Input: part model. Units: mm. Frame: model coordinates. A direction names the side the tool comes from. Give positions to 0.01 mm unless a question says otherwise; leave off trailing zeros. Write each loop counter-clockwise with the first axis right and the second up, starting at its lowest first coordinate (ties: lowest second). Pieces come first, ordered by that corner, then holes. Notation, with made-up numbers: (-30, -20) - (1, -20) arc R30 ccw to (1, 9) - close; hole circle Ø8 at (82, 38.5). An arc over 180 degrees is marked (long way). Answer as CSV lines item,"result". Start each with the question number.
from build123d import *

# Parameters (mm, degrees)
SKETCH056_R     = 1.05
PAD039_DEPTH    = 2
SKETCH057_W     = 10
SKETCH057_H     = 4
PAD040_DEPTH    = 10
SKETCH058_R     = 1.75
POCKET009_DEPTH = 4.001


with BuildPart() as part:
    # Sketch056 → Pad039 (new body)
    with BuildSketch(Plane.YZ):
        Polygon((-21.25, 67), (-16.25, 67), (-16.25, 39), (16.25, 39), (16.25, 67), (21.25, 67), (21.25, 34), (5, 34), (5, 4), (-5, 4), (-5, 34), (-21.25, 34), align=None)
        with Locations((-18.75, 60.75)):
            Circle(SKETCH056_R, mode=Mode.SUBTRACT)
        with Locations((-18.75, 45.25)):
            Circle(SKETCH056_R, mode=Mode.SUBTRACT)
        with Locations((18.75, 45.25)):
            Circle(SKETCH056_R, mode=Mode.SUBTRACT)
        with Locations((18.75, 60.75)):
            Circle(SKETCH056_R, mode=Mode.SUBTRACT)
    extrude(amount=PAD039_DEPTH)

    # Sketch057 (on Face18 of Pad039) → Pad040 (join)
    with BuildSketch(Plane.YZ.offset(2)):
        with Locations((0, 6)):
            Rectangle(SKETCH057_W, SKETCH057_H)
    extrude(amount=PAD040_DEPTH)

    # Sketch058 (on Face19 of Pad040) → Pocket009 (cut, through all)
    with BuildSketch(Plane(origin=(0, 0, 8), x_dir=(0, -1, 0), z_dir=(0, 0, 1))):
        with Locations((0, 7)):
            Circle(SKETCH058_R)
    extrude(amount=-POCKET009_DEPTH, mode=Mode.SUBTRACT)


with BuildPart() as part_1:
    # Body013 placement: moved
    add(part.part.moved(Location((41, 0, 0))))


solid = part_1.part
1) Contact query for flat-ended pins moving along their axis: P1, Ø1, axis at x = 42, y = -16.5, coming from the -Z side; P2, Ø5, axis at x = 44, z = 25.5, coming from the +Y side; P3, Ø1, axis at x = 42, y = -3, coming from the +Z side. Output: stop coordinate, or through.
2) Cut plane A-A on z = 58.5. Output: boundary loops of the cut face in (x, y).
3) Reachability of faces 5 (the flat face through (46, 0, 8)), 6 (the flat face through (42, 13, 34)), 7 (the flat face through (42, -13, 34)) from +Z, -Z, +X, -X, +Y, -Y: full face, straight path, thin tool, end or side. Return the list, or none.
4) Pull-direction query (Y, two-part tool) for faces 1 (the flat face through (42, -19, 67)), 2 (the flat face through (42, 0, 39)), 3 (the flat face through (42, -21.25, 50)), 4 (the flat face through (42, 21.25, 51)); classes: +Y half, -Y half, draft (parallel to the pull), parting line (faces both ways), or undercut.
5) Material intervals for line 1 (Z direction, x = 41.5, y = 18.75); line 2 (Y direction, x = 51.5, z = 7); line 3 (Z direction, x = 42.75, y = -9.5), sorted ascending. Write a range as from..to.
6) Cut plane B-B on y = 0. Output: boundary loops of the cut face in (x, z).
7) Cut plane C-C on y = 18.75. Output: boundary loops of the cut face in (x, z).
8) Cut plane D-D on x = 47. Output: boundary loops of the cut face in (y, z), and give its area (3 significant figures).
Numbers:
1,P1,"stops at z = 34"
1,P2,"stops at y = 5"
1,P3,"stops at z = 39"
2,outline,"(41, -21.25) - (43, -21.25) - (43, -16.25) - (41, -16.25) - close; (41, 16.25) - (43, 16.25) - (43, 21.25) - (41, 21.25) - close"
3,face 5,"+Z, +X, +Y, -Y"
3,face 6,"-Z, +X, -X, +Y"
3,face 7,"-Z, +X, -X, -Y"
4,face 1,"draft"
4,face 2,"undercut"
4,face 3,"-Y half"
4,face 4,"+Y half"
5,line 1,"z = 34..44.2, 46.3..59.7, 61.8..67"
5,line 2,"y = -5..5"
5,line 3,"z = 34..39"
6,outline,"(41, 4) - (46.25, 4) - (46.25, 8) - (43, 8) - (43, 39) - (41, 39) - close; (49.75, 4) - (53, 4) - (53, 8) - (49.75, 8) - close"
7,outline,"(41, 34) - (43, 34) - (43, 44.2) - (41, 44.2) - close; (41, 46.3) - (43, 46.3) - (43, 59.7) - (41, 59.7) - close; (41, 61.8) - (43, 61.8) - (43, 67) - (41, 67) - close"
8,outline,"(-5, 4) - (-1.44, 4) - (-1.44, 8) - (-5, 8) - close; (1.44, 4) - (5, 4) - (5, 8) - (1.44, 8) - close"
8,area,"28.5 mm²"
